```python
from build123d import *

# Parameters (mm, degrees)
SKETCH1_R           = 2.286
BOSS_EXTRUDE1_DEPTH = 9.525
SKETCH3_W           = 19.05
SKETCH3_H           = 10.795
CUT_EXTRUDE1_DEPTH  = 42.162500531
FILLET1_R           = 3.81


with BuildPart() as part:
    # Sketch1 → Boss-Extrude1 (new, symmetric)
    with BuildSketch(Plane(origin=(0, 0, 0), x_dir=(1, 0, 0), z_dir=(0, 1, 0))):
        with BuildLine():
            Line((33.655, -5.08), (-33.655, -5.08))
            ThreePointArc((-33.655, -5.08), (-38.735, 0), (-33.655, 5.08))
            Line((-33.655, 5.08), (33.655, 5.08))
            ThreePointArc((33.655, 5.08), (38.735, 0), (33.655, -5.08))
        make_face()
        with Locations(Location((0, 0, 0), (0, 0, 90))):
            Circle(SKETCH1_R, mode=Mode.SUBTRACT)
        with BuildLine():
            Line((33.655, -2.286), (29.845, -2.286))
            ThreePointArc((29.845, -2.286), (27.559, 0), (29.845, 2.286))
            Line((29.845, 2.286), (33.655, 2.286))
            ThreePointArc((33.655, 2.286), (35.941, 0), (33.655, -2.286))
        make_face(mode=Mode.SUBTRACT)
        with BuildLine():
            Line((-33.655, 2.286), (-29.845, 2.286))
            ThreePointArc((-29.845, 2.286), (-27.559, 0), (-29.845, -2.286))
            Line((-29.845, -2.286), (-33.655, -2.286))
            ThreePointArc((-33.655, -2.286), (-35.941, 0), (-33.655, 2.286))
        make_face(mode=Mode.SUBTRACT)
    extrude(amount=BOSS_EXTRUDE1_DEPTH, both=True)

    # Sketch3 → Cut-Extrude1 (cut, through all)
    with BuildSketch(Plane.XY.offset(5.08)):
        with Locations((-29.21, 0)):
            Rectangle(SKETCH3_W, SKETCH3_H)
        Rectangle(SKETCH3_W, SKETCH3_H)
        with Locations((29.21, 0)):
            Rectangle(SKETCH3_W, SKETCH3_H)
    extrude(amount=-CUT_EXTRUDE1_DEPTH, mode=Mode.SUBTRACT)

    # Fillet1
    fillet1_edges = [part.edges().sort_by_distance(p)[0] for p in [
        (19.685, 0, -5.08),
        (19.685, 0, 5.08),
        (-19.685, 0, 5.08),
        (-19.685, 0, -5.08),
        (-9.525, 0, -5.08),
        (9.525, 0, -5.08),
        (-9.525, 0, 5.08),
        (9.525, 0, 5.08),
    ]]
    fillet(fillet1_edges, radius=FILLET1_R)


solid = part.part
```
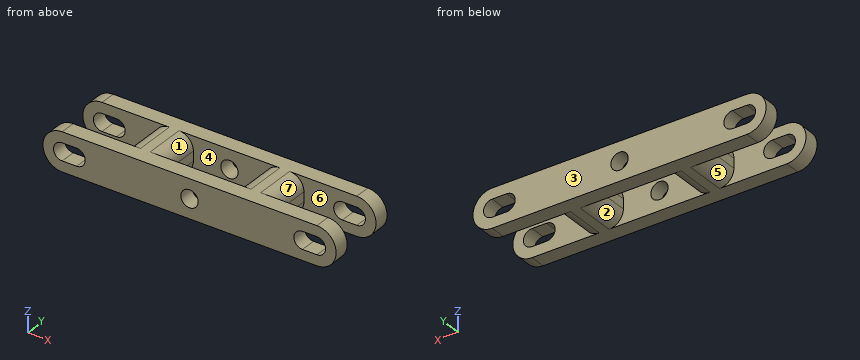
For this review, take the finished solid that the model builds, in its own axes (mm). Face numbers are marked on the shaded views. A direction names the side the tool comes from. Round coordinates to 2 decimals unless told otherwise and drop trailing zeros. Write each loop counter-clockwise with the first axis right and the second up, starting at its lowest first coordinate (ties: lowest second). Pieces come first, ordered by that corner, then holes. Notation, with made-up numbers: (-30.5, 81) - (-8.5, 81) arc R24 cw to (-8.5, 104) - close; hole circle Ø4 at (40.5, 30). An arc over 180 degrees is marked (long way). Put each result on its own line as item: value.
Q1. Insertion check: pin 1 Ø4 at (y, z) = (1, 1) entering from +X (3 decimals); pin 2 Ø1.5 at (y, z) = (1.5, 0.5) entering from -X (3 decimals); pin 3 Ø3 at (y, z) = (-7, 0.5) entering from +X (3 decimals); pin 4 Ø3.5 at (x, z) = (0, 0) entering from -Y. Each pin has a flat end and moves straight along its axis. Give the tip position at first contact, or say it passes through.
Solved:
pin 1: stops at x = 19.685
pin 2: stops at x = -19.685
pin 3: stops at x = 38.735
pin 4: passes through
Q2. Machinability: for the marked faces 1, 2 and 3, which of the approach directions +Z, -Z, +X, -X, +Y, -Y give a long, thin tool a straight path to every point of the face, cutting with its end or side? Answer none if there is none.
Solved:
face 1: +Z
face 2: -Z
face 3: +Z, -Z, +X, -X, +Y
Q3. We need section C-C (y = 1.75). Give the boundary of the cut face in (x, z) (3 decimals).
Solved:
outline: (-19.685, -1.27) arc R3.81 ccw to (-15.875, -5.08) - (-13.335, -5.08) arc R3.81 ccw to (-9.525, -1.27) - (-9.525, 1.27) arc R3.81 ccw to (-13.335, 5.08) - (-15.875, 5.08) arc R3.81 ccw to (-19.685, 1.27) - close; (9.525, -1.27) arc R3.81 ccw to (13.335, -5.08) - (15.875, -5.08) arc R3.81 ccw to (19.685, -1.27) - (19.685, 1.27) arc R3.81 ccw to (15.875, 5.08) - (13.335, 5.08) arc R3.81 ccw to (9.525, 1.27) - close
Q4. Mouldability with a two-part tool opening along X and no side actions: class the marked faces 4, 5, 6 and 7 as released by +X, released by -X, zero draft, split by the parting line, or undercut.
Solved:
face 4: undercut
face 5: released by -X
face 6: zero draft
face 7: released by +X
Q5. We need section B-B (x = 0). Give the boundary of the cut face in (y, z) (1 decimal).
Solved:
outline: (-9.5, -5.1) - (-5.4, -5.1) - (-5.4, -2.3) - (-9.5, -2.3) - close; (-9.5, 2.3) - (-5.4, 2.3) - (-5.4, 5.1) - (-9.5, 5.1) - close; (5.4, -5.1) - (9.5, -5.1) - (9.5, -2.3) - (5.4, -2.3) - close; (5.4, 2.3) - (9.5, 2.3) - (9.5, 5.1) - (5.4, 5.1) - close
Q6. Wall thickness on probe 1 along X at (y, z) = (-7.95, 0) (3 decimals); probe 2 along Y at (x, z) = (6.5, -3.5) (1 decimal); probe 3 along X at (y, z) = (-7, 1.5): over which ranges is each line inside the solid? List them lowest first.
Solved:
probe 1: x = -38.735 to -35.941, -27.559 to -2.286, 2.286 to 27.559, 35.941 to 38.735
probe 2: y = -9.5 to -5.4, 5.4 to 9.5
probe 3: x = -38.51 to -35.38, -28.12 to -1.73, 1.73 to 28.12, 35.38 to 38.51
Q7. We need section D-D (z = -3.25). Give the boundary of the cut face in (x, y) (1 decimal), and give its area (4 significant figures).
Solved:
outline: (-37.6, -9.5) - (37.6, -9.5) - (37.6, -5.4) - (19.1, -5.4) - (19.1, 5.4) - (37.6, 5.4) - (37.6, 9.5) - (-37.6, 9.5) - (-37.6, 5.4) - (-19.1, 5.4) - (-19.1, -5.4) - (-37.6, -5.4) - close; hole (-10.1, -5.4) - (10.1, -5.4) - (10.1, 5.4) - (-10.1, 5.4) - close
area: 815.5 mm2
Q8. We need section A-A (y = -6.5). Give the boundary of the cut face in (x, z) (3 decimals), and give its area (3 significant figures).
Solved:
outline: (-33.655, -5.08) - (33.655, -5.08) arc R5.08 ccw to (33.655, 5.08) - (-33.655, 5.08) arc R5.08 ccw to start; hole (-33.655, -2.286) - (-29.845, -2.286) arc R2.286 ccw to (-29.845, 2.286) - (-33.655, 2.286) arc R2.286 ccw to start; hole circle Ø4.572 at (0, 0); hole (29.845, -2.286) - (33.655, -2.286) arc R2.286 ccw to (33.655, 2.286) - (29.845, 2.286) arc R2.286 ccw to start
area: 681 mm2
